Source: CAD feature listing. Evaluate the final solid. Frame: model axes, mm. Face numbers are marked on the shaded views. A direction names the side the tool comes from. Give positions to 0.01 mm unless a question says otherwise; leave off trailing zeros. Write each loop counter-clockwise with the first axis right and the second up, starting at its lowest first coordinate (ties: lowest second). Pieces come first, ordered by that corner, then holes.
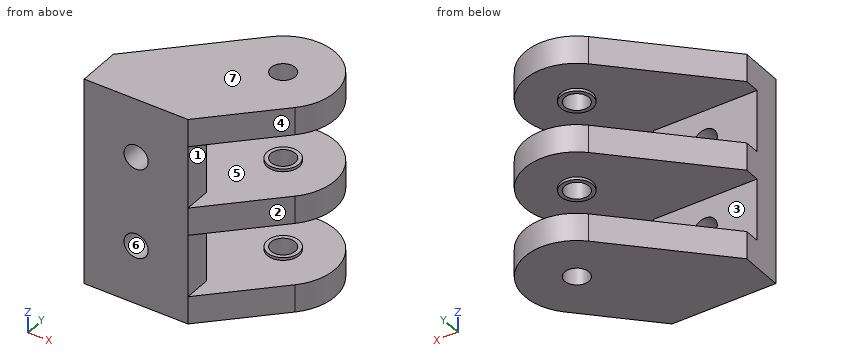
```python
from build123d import *

# Parameters (mm, degrees)
F0_R      = 1.75
F1_DEPTH  = 30
F2_W      = 23.070765
F2_H      = 9
F2_W_2    = 27.746933
F3_DEPTH  = 39.1
F4_W      = 2.213204
F4_H      = 16.336968
F5_DEPTH  = 500
F6_R      = 2.30465
F6_R_2    = 1.75
F7_DEPTH  = 0.4
F8_R      = 2.30465
F8_R_2    = 1.75
F9_DEPTH  = 0.4
F10_R     = 2.30465
F10_R_2   = 1.75
F11_DEPTH = 0.4
F12_R     = 2.30465
F12_R_2   = 1.75
F13_DEPTH = 0.4
F14_W     = 4
F14_H     = 9
F15_DEPTH = 6
F16_R     = 1.75
F17_DEPTH = 25


with BuildPart() as f1:
    # F0 (on Top) → F1 (new body)
    with BuildSketch(Plane.XY):
        with BuildLine():
            Line((-15.037711, -5.349152), (2.175493, -5.349152))
            Line((2.175493, -5.349152), (11.420161, 3.895517))
            ThreePointArc((11.420161, 3.895517), (11.420161, 14.502118), (0.813559, 14.502118))
            Line((0.813559, 14.502118), (-15.037711, -1.349152))
            Line((-15.037711, -1.349152), (-15.037711, -5.349152))
        make_face()
        with Locations((6.11686, 9.198817)):
            Circle(F0_R, mode=Mode.SUBTRACT)
    extrude(amount=F1_DEPTH)

    # F2 (on face) → F3 (cut)
    with BuildSketch(Plane(origin=(-15.037711, 0, 0), x_dir=(0, -1, 0), z_dir=(-1, 0, 0))):
        with Locations((-10.18623, 8.5)):
            Rectangle(F2_W, F2_H)
        with Locations((-12.524314, 21.5)):
            Rectangle(F2_W_2, F2_H)
    extrude(amount=-F3_DEPTH, mode=Mode.SUBTRACT)

    # F4 (on face) → F5 (cut)
    with BuildSketch(Plane.XY.offset(30)):
        with Locations((-13.931109, 2.819332)):
            Rectangle(F4_W, F4_H)
    extrude(amount=-F5_DEPTH, mode=Mode.SUBTRACT)

    # F6 (on face) → F7 (join)
    with BuildSketch(Plane(origin=(0, 0, 13), x_dir=(1, 0, 0), z_dir=(0, 0, -1))):
        with Locations((6.11686, -9.198817)):
            Circle(F6_R)
        with Locations((6.11686, -9.198817)):
            Circle(F6_R_2, mode=Mode.SUBTRACT)
    extrude(amount=F7_DEPTH)

    # F8 (on face) → F9 (join)
    with BuildSketch(Plane(origin=(0, 0, 26), x_dir=(1, 0, 0), z_dir=(0, 0, -1))):
        with Locations((6.11686, -9.198817)):
            Circle(F8_R)
        with Locations((6.11686, -9.198817)):
            Circle(F8_R_2, mode=Mode.SUBTRACT)
    extrude(amount=F9_DEPTH)

    # F10 (on face) → F11 (join)
    with BuildSketch(Plane.XY.offset(17)):
        with Locations((6.11686, 9.198817)):
            Circle(F10_R)
        with Locations((6.11686, 9.198817)):
            Circle(F10_R_2, mode=Mode.SUBTRACT)
    extrude(amount=F11_DEPTH)

    # F12 (on face) → F13 (join)
    with BuildSketch(Plane.XY.offset(4)):
        with Locations((6.11686, 9.198817)):
            Circle(F12_R)
        with Locations((6.11686, 9.198817)):
            Circle(F12_R_2, mode=Mode.SUBTRACT)
    extrude(amount=F13_DEPTH)

    # F14 (on face) → F15 (cut)
    with BuildSketch(Plane.XZ.offset(5.349152)):
        with Locations((4.175493, 8.5)):
            Rectangle(F14_W, F14_H)
        with Locations((4.175493, 21.5)):
            Rectangle(F14_W, F14_H)
    extrude(amount=-F15_DEPTH, mode=Mode.SUBTRACT)

    # F16 (on face) → F17 (cut)
    with BuildSketch(Plane(origin=(0, -1.349152, 0), x_dir=(-1, 0, 0), z_dir=(0, 1, 0))):
        with Locations((5.324507, 21.5)):
            Circle(F16_R)
        with Locations((5.324507, 8.5)):
            Circle(F16_R)
    extrude(amount=-F17_DEPTH, mode=Mode.SUBTRACT)


solid = f1.part
```
1. Line query: L1, parallel to Z at x = 1.25, y = 2.25; L2, parallel to Y at x = -5.75, z = 11.5; L3, parallel to Y at x = 11, z = 15.5. Output: solid intervals per line, ascending.
2. Access query for the marked faces 1, 2 and 3. Directions: +Z, -Z, +X, -X, +Y, -Y. A direction counts if a zero-diameter tool reaches every point of the face in a straight line with its end or side. Return the directions, or none.
3. Cut plane A-A, the plane z = 21.5. Return the cut outline in (x, y), then the cut area to 3 significant figures.
4. Contact query for flat-ended pins moving along their axis: P1, Ø4.5, axis at y = -2.5, z = 8.5, coming from the +X side; P2, Ø2.5, axis at x = -2, z = 7, coming from the +Y side; P3, Ø1, axis at x = -6.5, z = 16, coming from the +Y side. Output: stop coordinate, or through.
5. Mould query, pull axis Z, two halves, no side actions, for the marked faces 4, 5, 6 and 7. Classes: +Z half, -Z half, draft (parallel to the pull), parting line (faces both ways), or undercut.
6. Cut plane C-C, the plane y = -1.75. Return the cut outline in (x, z), then the cut area to 3 significant figures.
7. Cut plane B-B, the plane y = 1.25. Return the cut outline in (x, z).
8. Cut plane D-D, the plane x = -2.5. Return the cut outline in (y, z), then the cut area to 3 significant figures.
Response values:
1. L1: z = 0 to 4, 13 to 17, 26 to 30
1. L2: y = -5.35 to -1.35
1. L3: y = 3.48 to 14.89
2. face 1: +X, +Y, -Y
2. face 2: +Z, -Z, +X, -Y
2. face 3: +X, -X, +Y
3. outline: (-12.82, -5.35) - (-7.07, -5.35) - (-7.07, -1.35) - (-12.82, -1.35) - close; (-3.57, -5.35) - (2.18, -5.35) - (2.18, -1.35) - (-3.57, -1.35) - close
3. area: 46.0 mm2
4. P1: stops at x = 2.18
4. P2: stops at y = -1.35
4. P3: stops at y = 7.69
5. face 4: draft
5. face 5: undercut
5. face 6: undercut
5. face 7: +Z half
6. outline: (-12.82, 0) - (5.77, 0) - (5.77, 4) - (2.18, 4) - (2.18, 13) - (5.77, 13) - (5.77, 17) - (2.18, 17) - (2.18, 26) - (5.77, 26) - (5.77, 30) - (-12.82, 30) - close; hole circle Ø3.5 at (-5.32, 8.5); hole circle Ø3.5 at (-5.32, 21.5)
6. area: 474 mm2
7. outline: (-12.44, 0) - (8.77, 0) - (8.77, 4) - (-12.44, 4) - close; (-12.44, 13) - (8.77, 13) - (8.77, 17) - (-12.44, 17) - close; (-12.44, 26) - (8.77, 26) - (8.77, 30) - (-12.44, 30) - close
8. outline: (-5.35, 0) - (11.19, 0) - (11.19, 4) - (-1.35, 4) - (-1.35, 13) - (11.19, 13) - (11.19, 17) - (-1.35, 17) - (-1.35, 26) - (11.19, 26) - (11.19, 30) - (-5.35, 30) - close
8. area: 270 mm2
